The model under review builds one solid part; all positions refer to its coordinate system, in mm. A direction names the side the tool comes from. Coordinates: 2 decimals unless noted, no trailing zeros. Order: outer loops, then holes, each group sorted by start corner. A loop starts at its lowest first (then second) coordinate and runs counter-clockwise, first axis right, second up.
from build123d import *

# Parameters (mm, degrees)
SKETCH_1_R           = 4
SKETCH_1_R_2         = 15
EXTRUDE_2_DEPTH      = 10
SKETCH_2_W           = 48
SKETCH_2_H           = 4
CUT_EXTRUDE_3_DEPTH  = 68.453687816
CUT_EXTRUDE_4_DEPTH  = 68.453687816
SKETCH_4_W           = 48
SKETCH_4_H           = 4
EXTRUDE_3_DEPTH      = 10
SKETCH_5_W           = 10
SKETCH_5_H           = 4
EXTRUDE_4_DEPTH      = 100
SKETCH_6_W           = 15
SKETCH_6_H           = 10
CUT_EXTRUDE_5_DEPTH  = 100
SKETCH_7_R           = 2.5
CUT_EXTRUDE_14_DEPTH = 117.404467268
SKETCH_11_R          = 4
CUT_EXTRUDE_15_DEPTH = 68.45368795
SKETCH_12_R          = 15
EXTRUDE_5_DEPTH      = 10
SKETCH_14_W          = 100
SKETCH_14_H          = 10
EXTRUDE_6_DEPTH      = 30
SKETCH_15_R          = 2.5
CUT_EXTRUDE_16_DEPTH = 117.40446729
SKETCH_16_R          = 4
CUT_EXTRUDE_17_DEPTH = 68.45368795
SKETCH_17_W          = 15
SKETCH_17_H          = 30
EXTRUDE_7_DEPTH      = 10
SKETCH_18_R          = 2.5
CUT_EXTRUDE_18_DEPTH = 132.244047492
CUT_EXTRUDE_19_DEPTH = 132.244047591


with BuildPart() as part:
    # 草图1 → 凸台-拉伸2 (new body)
    # profile 1 of 3: a face of its own
    with BuildSketch(Plane.XY):
        with BuildLine():
            Line((50.00000004, 15), (-50, 15))
            ThreePointArc((-50, 15), (-39.393398282, 10.606601718), (-35, 0))
            ThreePointArc((-35, 0), (-39.393398282, -10.606601718), (-50, -15))
            Line((-50, -15), (50, -15))
            ThreePointArc((50, -15), (35, 2e-08), (50.00000004, 15))
        make_face()
        Circle(SKETCH_1_R, mode=Mode.SUBTRACT)
    # profile 2 of 3: a face of its own
    with BuildSketch(Plane.XY):
        with Locations((-50, 0)):
            Circle(SKETCH_1_R_2)
    # profile 3 of 3: a face of its own
    with BuildSketch(Plane.XY):
        with Locations((50, 0)):
            Circle(SKETCH_1_R_2)
    extrude(amount=EXTRUDE_2_DEPTH)

    # 草图2 → 切除-拉伸3 (cut, through all)
    with BuildSketch(Plane.XY.offset(10)):
        with Locations((26, 10)):
            Rectangle(SKETCH_2_W, SKETCH_2_H)
        with Locations((-26, 10)):
            Rectangle(SKETCH_2_W, SKETCH_2_H)
        with Locations((-26, -10)):
            Rectangle(SKETCH_2_W, SKETCH_2_H)
        with Locations((26, -10)):
            Rectangle(SKETCH_2_W, SKETCH_2_H)
    extrude(amount=-CUT_EXTRUDE_3_DEPTH, mode=Mode.SUBTRACT)

    # 草图3 → 切除-拉伸4 (cut, through all)
    with BuildSketch(Plane.XY.offset(10)):
        with BuildLine():
            Line((-3.464101615, 2), (-50, 2))
            Line((-50, 2), (-50, 0))
            Line((-50, 0), (-4, 0))
            ThreePointArc((-4, 0), (-3.863703305, 1.03527618), (-3.464101615, 2))
        make_face()
        with BuildLine():
            Line((-4, 0), (-50, 0))
            Line((-50, 0), (-50, -2))
            Line((-50, -2), (-3.464101615, -2))
            ThreePointArc((-3.464101615, -2), (-3.863703305, -1.03527618), (-4, 0))
        make_face()
        with BuildLine():
            Line((50, 0), (4, 0))
            ThreePointArc((4, 0), (3.863703305, -1.03527618), (3.464101615, -2))
            Line((3.464101615, -2), (50, -2))
            Line((50, -2), (50, 0))
        make_face()
        with BuildLine():
            Line((50, 2), (3.464101615, 2))
            ThreePointArc((3.464101615, 2), (3.863703305, 1.03527618), (4, 0))
            Line((4, 0), (50, 0))
            Line((50, 0), (50, 2))
        make_face()
    extrude(amount=-CUT_EXTRUDE_4_DEPTH, mode=Mode.SUBTRACT)

    # 草图4 → 凸台-拉伸3 (add)
    with BuildSketch(Plane.XY.offset(10)):
        with Locations((26, 10)):
            Rectangle(SKETCH_4_W, SKETCH_4_H)
        with Locations((26, -10)):
            Rectangle(SKETCH_4_W, SKETCH_4_H)
        with Locations((-26, 10)):
            Rectangle(SKETCH_4_W, SKETCH_4_H)
        with Locations((-26, -10)):
            Rectangle(SKETCH_4_W, SKETCH_4_H)
    extrude(amount=-EXTRUDE_3_DEPTH)

    # 草图5 → 凸台-拉伸4 (add)
    with BuildSketch(Plane(origin=(-50, 0, 0), x_dir=(0, 0, -1), z_dir=(1, 0, 0))):
        with Locations((-5, 0)):
            Rectangle(SKETCH_5_W, SKETCH_5_H)
    extrude(amount=EXTRUDE_4_DEPTH)

    # 草图6 → 切除-拉伸5 (cut)
    with BuildSketch(Plane.XZ.offset(15)):
        with Locations((-57.5, 5)):
            Rectangle(SKETCH_6_W, SKETCH_6_H)
    extrude(amount=-CUT_EXTRUDE_5_DEPTH, mode=Mode.SUBTRACT)

    # 草图7 → 切除-拉伸14 (cut, through all)
    with BuildSketch(Plane.ZY.offset(50)):
        with Locations((5, 0)):
            Circle(SKETCH_7_R)
    extrude(amount=-CUT_EXTRUDE_14_DEPTH, mode=Mode.SUBTRACT)

    # 草图11 → 切除-拉伸15 (cut, through all)
    with BuildSketch(Plane.XY.offset(10)):
        Circle(SKETCH_11_R)
    extrude(amount=-CUT_EXTRUDE_15_DEPTH, mode=Mode.SUBTRACT)

    # 草图12 → 凸台-拉伸5 (add)
    with BuildSketch(Plane.XY.offset(10)):
        with Locations((-50, 0)):
            Circle(SKETCH_12_R)
    extrude(amount=-EXTRUDE_5_DEPTH)

    # 草图14 → 凸台-拉伸6 (add)
    with BuildSketch(Plane(origin=(0, 15, 0), x_dir=(1, 0, 0), z_dir=(0, 1, 0))):
        with Locations((0, -5)):
            Rectangle(SKETCH_14_W, SKETCH_14_H)
    extrude(amount=-EXTRUDE_6_DEPTH)

    # 草图15 → 切除-拉伸16 (cut, through all)
    with BuildSketch(Plane(origin=(50, 0, 0), x_dir=(0, 0, -1), z_dir=(1, 0, 0))):
        with Locations(Location((-5, 0, 0), (0, 0, 180))):
            Circle(SKETCH_15_R)
    extrude(amount=-CUT_EXTRUDE_16_DEPTH, mode=Mode.SUBTRACT)

    # 草图16 → 切除-拉伸17 (cut, through all)
    with BuildSketch(Plane.XY.offset(10)):
        Circle(SKETCH_16_R)
    extrude(amount=-CUT_EXTRUDE_17_DEPTH, mode=Mode.SUBTRACT)

    # 草图17 → 凸台-拉伸7 (add)
    with BuildSketch(Plane.XY.offset(10)):
        with Locations((57.5, 0)):
            Rectangle(SKETCH_17_W, SKETCH_17_H)
        with Locations((-57.5, 0)):
            Rectangle(SKETCH_17_W, SKETCH_17_H)
    extrude(amount=-EXTRUDE_7_DEPTH)

    # 草图18 → 切除-拉伸18 (cut, through all)
    with BuildSketch(Plane.ZY.offset(65)):
        with Locations((5, 0)):
            Circle(SKETCH_18_R)
    extrude(amount=-CUT_EXTRUDE_18_DEPTH, mode=Mode.SUBTRACT)

    # 草图19 → 切除-拉伸19 (cut, through all)
    with BuildSketch(Plane.ZY.offset(65)):
        with BuildLine():
            Line((10, 1.767766953), (6.767766953, 1.767766953))
            ThreePointArc((6.767766953, 1.767766953), (7.309698831, 0.956708581), (7.5, 0))
            ThreePointArc((7.5, 0), (7.309698831, -0.956708581), (6.767766953, -1.767766953))
            Line((6.767766953, -1.767766953), (10, -1.767766953))
            Line((10, -1.767766953), (10, 1.767766953))
        make_face()
    extrude(amount=-CUT_EXTRUDE_19_DEPTH, mode=Mode.SUBTRACT)


solid = part.part
(1) Consider section A-A (y = 0). Give the boundary of the cut face in (x, z), then the cut area to 3 significant figures.
(2) Insertion check: pin 1 Ø4.5 at (y, z) = (0, 5) entering from -X. The pin has a flat end and moves straight along its axis. Give the tip position at first contact, or say it passes through.
(3) Consider section C-C (x = 0). Give the boundary of the cut face in (y, z), then the cut area to 3 significant figures.
(4) Consider section D-D (x = 55.5). Give the boundary of the cut face in (y, z).
(5) Wall thickness on line 1 (Y direction, x = -11, z = 9); line 2 (Y direction, x = 0, z = 5.75); line 3 (Z direction, x = 23.5, y = 0): over which ranges is each line inside the solid? List them lowest first.
(6) Tool access review of faces 4 (the face through (-1, -8, 10)), 5 (the face through (34, 1.768, 8)): name each direction out of +Z, -Z, +X, -X, +Y, -Y from which nothing blocks a thin tool from reaching the whole face with its end or side.
(7) Consider section B-B (z = 5). Give the boundary of the cut face in (x, y), then the cut area to 3 significant figures.
(8) The part is to be moulded in two halves that separate along Z. For faces 1 (the face through (-1, -7, 0)), 2 (the face through (-35, 1.768, 8)), 3 (the face through (33.6, 0.1, 2.5)), say which applies: +Z half, -Z half, draft (parallel to the pull), parting line (faces both ways), or undercut.
Findings:
1. outline: (-65, 0) - (-4, 0) - (-4, 2.5) - (-65, 2.5) - close; (4, 0) - (65, 0) - (65, 2.5) - (4, 2.5) - close
1. area: 305 mm2
2. pin 1: passes through
3. outline: (-15, 0) - (-4, 0) - (-4, 10) - (-15, 10) - close; (4, 0) - (15, 0) - (15, 10) - (4, 10) - close
3. area: 220 mm2
4. outline: (-15, 0) - (15, 0) - (15, 10) - (1.77, 10) - (1.77, 6.77) arc R2.5 cw (long way) to (-1.77, 6.77) - (-1.77, 10) - (-15, 10) - close
5. line 1: y = -15 to -1.77, 1.77 to 15
5. line 2: y = -15 to -4, 4 to 15
5. line 3: z = 0 to 2.5
6. face 4: +Z, +X, -X, +Y, -Y
6. face 5: +Z, +X, -X
7. outline: (-65, -15) - (65, -15) - (65, -2.5) - (3.12, -2.5) arc R4 cw to (-3.12, -2.5) - (-65, -2.5) - close; (-65, 2.5) - (-3.12, 2.5) arc R4 cw to (3.12, 2.5) - (65, 2.5) - (65, 15) - (-65, 15) - close
7. area: 3,240 mm2
8. face 1: -Z half
8. face 2: draft
8. face 3: undercut
